```python
from build123d import *

# Parameters (mm, degrees)
F0_W      = 152.5348722935
F0_H      = 110.0516840816
F1_DEPTH  = 25.4
F2_W      = 59.8810613155
F2_H      = 41.0670798738
F3_DEPTH  = 25.4
F5_DEPTH  = 25.4
F6_W      = 3.5402644426
F6_H      = 4.0460177697
F7_DEPTH  = 25.4
F8_W      = 49.3959197775
F8_H      = 34.7048761323
F9_DEPTH  = 25.4
F10_W     = 41.6679419577
F10_H     = 25.9291101247
F11_DEPTH = 25.4
F12_W     = 34.0640768409
F12_H     = 21.1985725909
F13_DEPTH = 25.4
F14_W     = 29.7382287681
F14_H     = 16.7909711599
F15_DEPTH = 25.4
F16_W     = 26.2991152704
F16_H     = 14.3633615226
F16_W_2   = 22.8600006667
F16_H_2   = 10.3173442185
F17_DEPTH = 25.4
F18_W     = 26.2991152704
F18_H     = 14.3633615226
F18_W_2   = 22.4553988955
F18_H_2   = 10.1150441915
F18_W_3   = 14.3633633852
F18_H_3   = 4.6529192477
F18_W_4   = 8.4966383874
F18_H_4   = 1.4161076397
F19_DEPTH = 25.4
F20_W     = 21.8484961079
F20_H     = 9.9127423018
F21_DEPTH = 25.4
F22_W     = 14.8691139184
F22_H     = 9.9127423018
F23_DEPTH = 25.4
F24_W     = 8.8000879623
F24_H     = 4.8552211374
F25_DEPTH = 25.4
F26_W     = 27.6140682399
F26_H     = 29.4347768649
F26_W_2   = 9.7104460001
F26_H_2   = 15.1725648902
F26_W_3   = 27.3106172681
F26_H_3   = 26.7037190497
F26_W_4   = 11.2277008593
F26_H_4   = 11.5311481059
F26_W_5   = 3.9448663592
F26_H_5   = 7.5862845405
F26_W_6   = 4.2483173311
F26_H_6   = 5.7655721903
F27_DEPTH = 25.4
F28_DEPTH = 25.4
F30_DEPTH = 25.4


with BuildPart() as f1:
    # F0 (on Front) → F1 (new body)
    with BuildSketch(Plane.XZ):
        with Locations((0.2022981644, 20.7358412445)):
            Rectangle(F0_W, F0_H)
    extrude(amount=F1_DEPTH)

    # F2 (on face) → F3 (join)
    with BuildSketch(Plane.XZ.offset(25.4)):
        with Locations((-10.3847794235, 22.6576993009)):
            Rectangle(F2_W, F2_H)
    extrude(amount=F3_DEPTH)

    # F4 (on face) → F5 (cut)
    with BuildSketch(Plane(origin=(-40.3253100812, 0, 0), x_dir=(0, -1, 0), z_dir=(-1, 0, 0))):
        Polygon((35.9776653349, 34.7957536578), (25.4, 34.7957536578), (25.4, 28.1198229641), (30.6888326675, 28.1198229641), (35.9776653349, 28.1198229641), align=None)
    extrude(amount=-F5_DEPTH, mode=Mode.SUBTRACT)

    # F6 (on face) → F7 (cut)
    with BuildSketch(Plane(origin=(-40.3253100812, 0, 0), x_dir=(0, -1, 0), z_dir=(-1, 0, 0))):
        with Locations((39.2070347443, 17.6001775544)):
            Rectangle(F6_W, F6_H)
        with Locations((39.2070347443, 13.5541597847)):
            Rectangle(F6_W, F6_H)
        with Locations((42.7472991869, 13.5541597847)):
            Rectangle(F6_W, F6_H)
        with Locations((42.7472991869, 17.6001775544)):
            Rectangle(F6_W, F6_H)
    extrude(amount=-F7_DEPTH, mode=Mode.SUBTRACT)

    # F8 (on face) → F9 (join)
    with BuildSketch(Plane.XZ.offset(50.8)):
        with Locations((-10.1041528396, 22.9534148239)):
            Rectangle(F8_W, F8_H)
    extrude(amount=F9_DEPTH)

    # F10 (on face) → F11 (join)
    with BuildSketch(Plane.XZ.offset(76.2)):
        with Locations((-10.1783443242, 24.4610188529)):
            Rectangle(F10_W, F10_H)
    extrude(amount=F11_DEPTH)

    # F12 (on face) → F13 (join)
    with BuildSketch(Plane.XZ.offset(101.6)):
        with Locations((-10.288214311, 23.9018974826)):
            Rectangle(F12_W, F12_H)
    extrude(amount=F13_DEPTH)

    # F14 (on face) → F15 (join)
    with BuildSketch(Plane.XZ.offset(127)):
        with Locations((-10.2836284786, 23.8715037704)):
            Rectangle(F14_W, F14_H)
    extrude(amount=F15_DEPTH)

    # F16 (on face) → F17 (join)
    with BuildSketch(Plane.XZ.offset(152.4)):
        with Locations((-10.3847794235, 25.085308589)):
            Rectangle(F16_W, F16_H)
        with Locations((-10.6882309483, 25.489911437)):
            Rectangle(F16_W_2, F16_H_2, mode=Mode.SUBTRACT)
        with Locations((-10.6882309483, 25.489911437)):
            Rectangle(F16_W_2, F16_H_2)
    extrude(amount=F17_DEPTH)

    # F18 (on face) → F19 (join)
    with BuildSketch(Plane.XZ.offset(177.8)):
        with Locations((-10.3847794235, 25.085308589)):
            Rectangle(F18_W, F18_H)
        with Locations((-10.8905318339, 25.3887614235)):
            Rectangle(F18_W_2, F18_H_2, mode=Mode.SUBTRACT)
        with Locations((-10.8905318339, 25.3887614235)):
            Rectangle(F18_W_2, F18_H_2)
        Polygon((-2.0904429257, 22.3542470485), (-20.499823615, 22.3542470485), (-20.499823615, 28.8278758526), (-18.6791159213, 28.8278758526), (-4.3157525361, 28.8278758526), (-2.0904429257, 28.8278758526), align=None, mode=Mode.SUBTRACT)
        Polygon((-20.499823615, 28.8278758526), (-20.499823615, 22.3542470485), (-2.0904429257, 22.3542470485), (-2.0904429257, 28.8278758526), (-4.3157525361, 28.8278758526), (-4.3157525361, 24.1749566048), (-18.6791159213, 24.1749566048), (-18.6791159213, 28.8278758526), align=None)
        with Locations((-11.4974342287, 26.5014162287)):
            Rectangle(F18_W_3, F18_H_3)
        with Locations((-12.2054871172, 26.5014162287)):
            Rectangle(F18_W_4, F18_H_4, mode=Mode.SUBTRACT)
        with Locations((-12.2054871172, 26.5014162287)):
            Rectangle(F18_W_4, F18_H_4)
    extrude(amount=F19_DEPTH)

    # F20 (on face) → F21 (join)
    with BuildSketch(Plane.XZ.offset(203.2)):
        with Locations((-10.789381311, 25.2876104787)):
            Rectangle(F20_W, F20_H)
    extrude(amount=F21_DEPTH)

    # F22 (on face) → F23 (join)
    with BuildSketch(Plane.XZ.offset(228.6)):
        with Locations((-10.7893806417, 25.2876104787)):
            Rectangle(F22_W, F22_H)
    extrude(amount=F23_DEPTH)

    # F24 (on face) → F25 (join)
    with BuildSketch(Plane.XZ.offset(254)):
        with Locations((-10.4859292042, 25.4899105057)):
            Rectangle(F24_W, F24_H)
    extrude(amount=F25_DEPTH)

    # F26 (on face) → F27 (join)
    with BuildSketch(Plane(origin=(0, 0, 0), x_dir=(-1, 0, 0), z_dir=(0, 1, 0))):
        with Locations((47.5069899112, -1.9724336453)):
            Rectangle(F26_W, F26_H)
        with Locations((47.962166369, -1.2138050515)):
            Rectangle(F26_W_2, F26_H_2, mode=Mode.SUBTRACT)
        with Locations((47.3552644253, 51.8901776522)):
            Rectangle(F26_W_3, F26_H_3)
        with Locations((48.1138918549, 53.1039815396)):
            Rectangle(F26_W_4, F26_H_4, mode=Mode.SUBTRACT)
        Polygon((-4.8383618705, 12.1380519122), (-12.8798228689, 12.1380519122), (-21.5281862766, 12.1380519122), (-21.5281862766, -3.3379644156), (-4.8383618705, -3.3379644156), align=None)
        Polygon((-12.8798228689, 41.5728315711), (-21.5281862766, 41.5728315711), (-21.5281862766, 37.6279652119), (-21.5281862766, 12.1380519122), (-12.8798228689, 12.1380519122), align=None)
        Polygon((-4.2314594612, 41.5728315711), (-4.2314594612, 54.6212382615), (-21.5281862766, 54.6212382615), (-21.5281862766, 41.5728315711), (-12.8798228689, 41.5728315711), align=None)
        Polygon((-21.5281862766, 41.5728315711), (-21.5281862766, 54.6212382615), (-40.0387123227, 46.124599874), (-21.5281862766, 37.6279652119), align=None)
        with Locations((47.962166369, -1.2138050515)):
            Rectangle(F26_W_2, F26_H_2)
        with Locations((48.4173446894, -1.0620807297)):
            Rectangle(F26_W_5, F26_H_5, mode=Mode.SUBTRACT)
        Polygon((-21.5281862766, -3.3379644156), (-21.5281862766, 12.1380519122), (-40.0387123227, 4.5517692342), align=None)
        with Locations((48.1138918549, 53.1039815396)):
            Rectangle(F26_W_4, F26_H_4)
        with Locations((48.5690701753, 53.2557070255)):
            Rectangle(F26_W_6, F26_H_6, mode=Mode.SUBTRACT)
    extrude(amount=F27_DEPTH)

    # F28 (cut): faces of the model
    f28_faces = [f1.faces().sort_by_distance(p)[0] for p in [
        (-48.5690701753, 0, 53.2557070255),
        (-48.4173446894, 0, -1.0620807297),
    ]]
    extrude(f28_faces, amount=-F28_DEPTH, mode=Mode.SUBTRACT)

    # F29 (on face) → F30 (join)
    with BuildSketch(Plane.XZ.offset(25.4)):
        Polygon((26.4339819551, 50.2717718482), (47.270976007, 50.2717718482), (55.059555918, 50.2717718482), (55.059555918, 61.3983161747), (26.4339819551, 61.3983161747), align=None)
        Polygon((47.270976007, 50.2717718482), (47.270976007, -6.1701769009), (55.5653087795, -6.1701769009), (62.848135829, -6.1701769009), (62.848135829, 50.2717718482), (55.059555918, 50.2717718482), align=None)
        Polygon((47.270976007, -6.1701769009), (27.0408838987, -6.1701769009), (27.0408838987, -17.4990277737), (55.5653087795, -17.4990277737), (55.5653087795, -6.1701769009), align=None)
    extrude(amount=F30_DEPTH)


solid = f1.part
```
Check sheet for the modelled part. Datum: model origin and axes. Units: mm. A direction names the side the tool comes from. Round coordinates to 2 decimals unless told otherwise and drop trailing zeros. Order: outer loops, then holes, each group sorted by start corner. A loop starts at its lowest first (then second) coordinate and runs counter-clockwise, first axis right, second up. Notation, with made-up numbers: M 68.5,20.25 L 127.5,20.25 A21 cw 127.5,45.25 Z; hole C 23,52 d7. An arc over 180 degrees is marked long. Answer in a Markdown table with one row per item.
(1) Set-up check for faces 1 (the flat face through (41, -38, -17.499)), 2 (the flat face through (-40.325, -38, 22)), 3 (the flat face through (-47, 13, 65.242)), 4 (the flat face through (-46.445, 0, -1)), 5 (the flat face through (59, -38, 50.272)): record each of +Z, -Z, +X, -X, +Y, -Y from which the full face is reachable in a straight line by a thin tool's end or side.
Findings:
| item | result |
|---|---|
| face 1 | -Z, +X, -X, -Y |
| face 2 | +Z, -Z, -X, -Y |
| face 3 | +Z, +X, -X, +Y |
| face 4 | +Y, -Y |
| face 5 | +Z, +X, -Y |
(2) Draft check along Z on faces 6 (the flat face through (13, 13, -3.338)), 7 (the flat face through (47.271, -38, 22)), 8 (the flat face through (-18.224, -241, 25)), 9 (the flat face through (9, 13, 41.573)). Enter one of: +Z half, -Z half, draft (parallel to the pull), parting line (faces both ways), or undercut.
Findings:
| item | result |
|---|---|
| face 6 | -Z half |
| face 7 | undercut |
| face 8 | draft |
| face 9 | undercut |
(3) Section check C-C on y = -60.5. Record the boundary of the cut face in (x, z), plus the area to 3 significant figures.
Findings:
| item | result |
|---|---|
| outline | M -34.8,5.6 L 14.59,5.6 L 14.59,40.31 L -34.8,40.31 Z |
| area | 1,710 mm^2 |
(4) Section check B-B on x = 34. Record the boundary of the cut face in (y, z).
Findings:
| item | result |
|---|---|
| outline | M -50.8,-17.5 L -25.4,-17.5 L -25.4,-34.29 L 0,-34.29 L 0,1.98 L 25.4,1.98 L 25.4,7.03 L 0,7.03 L 0,43.35 L 25.4,43.35 L 25.4,48.9 L 0,48.9 L 0,75.76 L -25.4,75.76 L -25.4,61.4 L -50.8,61.4 L -50.8,50.27 L -25.4,50.27 L -25.4,-6.17 L -50.8,-6.17 Z |
(5) Material ranges on line 1 along X through (y, z) = (1, 53); line 2 along Y through (x, z) = (-24, 14.5); line 3 along Z through (x, y) = (-34, 10), recorded low to high. Write a range as from..to.
Findings:
| item | result |
|---|---|
| line 1 | x = -61.01..-50.69, -46.44..-33.7, 4.23..25.06 |
| line 2 | y = -127..-44.52, -37.44..0 |
| line 3 | z = -16.69..12.74, 38.54..65.24 |
(6) Gauge pin test, flat ends, axial feed: pin 1 (7.5 mm diameter, centred on x = -9.5, y = -94.5, fed in from -Z); pin 2 (2 mm diameter, centred on x = 52.5, z = -21.5, fed in from -Y); pin 3 (2.5 mm diameter, centred on x = -8.5, y = -269.5, fed in from -Z). Record the tip position at first contact, or that the pin passes through.
Findings:
| item | result |
|---|---|
| pin 1 | stops at z = 11.5 |
| pin 2 | stops at y = -25.4 |
| pin 3 | stops at z = 23.06 |
(7) Section check A-A on y = -199. Record the boundary of the cut face in (x, z).
Findings:
| item | result |
|---|---|
| outline | M -23.53,17.9 L 2.76,17.9 L 2.76,32.27 L -23.53,32.27 Z |
